Part model, mm, in its own coordinate system. A direction names the side the tool comes from. Coordinates: 2 decimals unless noted, no trailing zeros. Order: outer loops, then holes, each group sorted by start corner. A loop starts at its lowest first (then second) coordinate and runs counter-clockwise, first axis right, second up.
1) Wall check: L1, parallel to Y at x = -169.5, z = 124; L2, parallel to X at y = 385, z = 123.75; L3, parallel to Z at x = -194.65, y = 350.7. Give the ranges that are in metal, low to high.
2) Mould opens along Z. For faces 6 (the cylindrical face through (-194.72, 349, 132.57)), 7 (the flat face through (-177, 367, 117.5)), 8 (the cylindrical face through (-175.88, 368.68, 116.02)) say: +Z half, -Z half, draft (parallel to the pull), parting line (faces both ways), or undercut.
3) Pin check, flat tips, straight feed: pin 1 Ø5 at (x, z) = (-184, 130.5) entering from -Y; pin 2 Ø6 at (x, y) = (-160, 388.5) entering from +Z; pin 3 Ø8 at (x, z) = (-152, 126.5) entering from +Y; pin 4 Ø12 at (x, z) = (-172.5, 125) entering from -Y. Stop position of each tip, or through.
4) Tool access for faces 1 (the flat face through (-190, 363, 140.405)), 2 (the flat face through (-165, 379, 129.5)), 3 (the flat face through (-193, 386, 134)), 4 (the cylindrical face through (-153.436, 344.674, 121.049)), 5 (the flat face through (-191, 370.7, 134)): list every direction of +Z, -Z, +X, -X, +Y, -Y with a clear straight run to the whole face (end or side of a thin tool).
5) Cut at B-B (y = 383.7). Give the number of separate pieces and of enclosed holes in the cut face, and give its area (3 significant figures).
6) Cut at A-A (z = 127). List the corners of the cut face in (x, y), and give its area (3 significant figures).
```python
from build123d import *

# Parameters (mm, degrees)
BOX_W           = 55
BOX_H           = 95
BOX_DEPTH       = 10
SKETCH_R        = 2
POCKET_DEPTH    = 10
SKETCH001_R     = 2
POCKET001_DEPTH = 10
FILLET_R        = 1
PAD_DEPTH       = 20
CHAMFER_SIZE    = 20
CHAMFER001_SIZE = 20
SKETCH003_R     = 3
POCKET005_DEPTH = 6
SKETCH004_R     = 10
SKETCH004_R_2   = 2
PAD001_DEPTH    = 5
SKETCH005_W     = 3
SKETCH005_H     = 3
POCKET006_DEPTH = 5
SKETCH006_R     = 2.9
POCKET007_DEPTH = 3.5
SKETCH007_R     = 1.7
POCKET008_DEPTH = 5
SKETCH009_R     = 4.8
POCKET009_DEPTH = 9.5
CHAMFER002_SIZE = 1
CHAMFER003_SIZE = 1.5
SKETCH010_R     = 1.5
POCKET010_DEPTH = 8
SKETCH011_R     = 3
POCKET011_DEPTH = 1


with BuildPart() as part:
    # Box → Box (new body)
    with BuildSketch(Plane(origin=(-197, 315.2, 114.5), x_dir=(1, 0, 0), z_dir=(0, 0, 1))):
        with Locations((27.5, 47.5)):
            Rectangle(BOX_W, BOX_H)
    extrude(amount=BOX_DEPTH)

    # Sketch → Pocket (cut)
    with BuildSketch(Plane(origin=(-197, 315.2, 124.5), x_dir=(1, 0, 0), z_dir=(0, 0, 1))):
        with Locations((27.5, 26.5)):
            Circle(SKETCH_R)
        with Locations((27.5, 68.5)):
            Circle(SKETCH_R)
        Polygon((0, 74), (21.746137, 95), (0, 95), align=None)
        Polygon((33.253863, 95), (55, 95), (55, 74), align=None)
        Polygon((55, 21), (33.253863, 0), (55, 0), align=None)
        Polygon((0, 21), (0, 0), (21.746137, 0), align=None)
    extrude(amount=-POCKET_DEPTH, mode=Mode.SUBTRACT)

    # Sketch001 → Pocket001 (cut)
    with BuildSketch(Plane(origin=(-197, 315.2, 124.5), x_dir=(1, 0, 0), z_dir=(0, 0, 1))):
        with Locations((19.272759, 12.25)):
            Circle(SKETCH001_R)
        with Locations((19.272759, 40.75)):
            Circle(SKETCH001_R)
        with Locations((43.954483, 26.5)):
            Circle(SKETCH001_R)
        with Locations((19.272759, 54.25)):
            Circle(SKETCH001_R)
        with Locations((19.272759, 82.75)):
            Circle(SKETCH001_R)
        with Locations((43.954483, 68.5)):
            Circle(SKETCH001_R)
        with BuildLine():
            ThreePointArc((14.272759, 41.501336), (7.5, 26.5), (14.272759, 11.498664))
            Line((14.272759, 11.498664), (14.272759, 41.501336))
        make_face()
        with BuildLine():
            ThreePointArc((14.272759, 83.501336), (7.5, 68.5), (14.272759, 53.498664))
            Line((14.272759, 53.498664), (14.272759, 83.501336))
        make_face()
    extrude(amount=-POCKET001_DEPTH, mode=Mode.SUBTRACT)

    # Fillet
    fillet_edges = [part.edges().sort_by_distance(p)[0] for p in [
        (-182.727241, 326.698664, 119.5),
        (-175.727241, 355.95, 119.5),
        (-175.727241, 397.95, 119.5),
        (-182.727241, 356.701336, 119.5),
    ]]
    fillet(fillet_edges, radius=FILLET_R)

    # Sketch002 → Pad (new body)
    with BuildSketch(Plane(origin=(-197, 315.2, 124.5), x_dir=(1, 0, 0), z_dir=(0, 0, 1))):
        Polygon((4, 17.137245), (4, 31.5), (8, 31.5), (8, 39.5), (4, 39.5), (4, 45.5), (55, 45.5), (55, 49.5), (4, 49.5), (4, 55.5), (8, 55.5), (8, 63.5), (4, 63.5), (4, 77.862755), (0, 74), (0, 21), align=None)
    extrude(amount=PAD_DEPTH)

    # Chamfer
    chamfer_edges = [part.edges().sort_by_distance(p)[0] for p in [
        (-142, 362.7, 144.5),
    ]]
    chamfer(chamfer_edges, length=CHAMFER_SIZE)

    # Chamfer001
    chamfer001_edges = [part.edges().sort_by_distance(p)[0] for p in [
        (-162, 362.7, 144.5),
    ]]
    chamfer(chamfer001_edges, length=CHAMFER001_SIZE)

    # Sketch003 → Pocket005 (cut)
    with BuildSketch(Plane(origin=(-197, 315.2, 124.5), x_dir=(1, 0, 0), z_dir=(0, 0, 1))):
        with Locations((19.272759, 40.75)):
            Circle(SKETCH003_R)
        with Locations((19.272759, 12.25)):
            Circle(SKETCH003_R)
        with Locations((43.954483, 26.5)):
            Circle(SKETCH003_R)
        with Locations((19.272759, 54.25)):
            Circle(SKETCH003_R)
        with Locations((19.272759, 82.75)):
            Circle(SKETCH003_R)
        with Locations((43.954483, 68.5)):
            Circle(SKETCH003_R)
    extrude(amount=-POCKET005_DEPTH, mode=Mode.SUBTRACT)

    # Sketch004 → Pad001 (new body)
    with BuildSketch(Plane(origin=(-197, 315.2, 124.5), x_dir=(1, 0, 0), z_dir=(0, 0, 1))):
        with Locations((27.5, 68.5)):
            Circle(SKETCH004_R)
        with Locations((27.5, 68.5)):
            Circle(SKETCH004_R_2, mode=Mode.SUBTRACT)
        with Locations((27.5, 26.5)):
            Circle(SKETCH004_R)
        with Locations((27.5, 26.5)):
            Circle(SKETCH004_R_2, mode=Mode.SUBTRACT)
    extrude(amount=PAD001_DEPTH)

    # Sketch005 → Pocket006 (cut)
    with BuildSketch(Plane(origin=(-197, 360.7, 114.5), x_dir=(1, 0, 0), z_dir=(0, -1, 0))):
        with Locations((7.05428, 24.404704)):
            Rectangle(SKETCH005_W, SKETCH005_H)
        with Locations((20.05428, 24.404704)):
            Rectangle(SKETCH005_W, SKETCH005_H)
    extrude(amount=-POCKET006_DEPTH, mode=Mode.SUBTRACT)

    # Sketch006 → Pocket007 (cut)
    with BuildSketch(Plane(origin=(-189, 315.2, 114.5), x_dir=(0, 1, 0), z_dir=(1, 0, 0))):
        with Locations((35.5, 18)):
            Circle(SKETCH006_R)
        with Locations((59.5, 18)):
            Circle(SKETCH006_R)
    extrude(amount=-POCKET007_DEPTH, mode=Mode.SUBTRACT)

    # Sketch007 → Pocket008 (cut)
    with BuildSketch(Plane(origin=(-192.5, 315.2, 114.5), x_dir=(0, 1, 0), z_dir=(1, 0, 0))):
        with Locations((35.5, 18)):
            Circle(SKETCH007_R)
        with Locations((59.5, 18)):
            Circle(SKETCH007_R)
    extrude(amount=-POCKET008_DEPTH, mode=Mode.SUBTRACT)

    # Sketch009 → Pocket009 (cut)
    with BuildSketch(Plane(origin=(-197, 315.2, 129.5), x_dir=(1, 0, 0), z_dir=(0, 0, 1))):
        with Locations((27.5, 26.5)):
            Circle(SKETCH009_R)
        with Locations((27.5, 68.5)):
            Circle(SKETCH009_R)
    extrude(amount=-POCKET009_DEPTH, mode=Mode.SUBTRACT)

    # Chamfer002
    chamfer002_edges = [part.edges().sort_by_distance(p)[0] for p in [
        (-174.3, 383.7, 129.5),
        (-174.3, 341.7, 129.5),
    ]]
    chamfer(chamfer002_edges, length=CHAMFER002_SIZE)

    # Chamfer003
    chamfer003_edges = [part.edges().sort_by_distance(p)[0] for p in [
        (-171.5, 341.7, 120),
        (-171.5, 383.7, 120),
    ]]
    chamfer(chamfer003_edges, length=CHAMFER003_SIZE)

    # Sketch010 → Pocket010 (cut)
    with BuildSketch(Plane(origin=(-142, 315.2, 114.5), x_dir=(0, 1, 0), z_dir=(1, 0, 0))):
        with Locations((30, 5)):
            Circle(SKETCH010_R)
        with Locations((65, 5)):
            Circle(SKETCH010_R)
    extrude(amount=-POCKET010_DEPTH, mode=Mode.SUBTRACT)

    # Sketch011 → Pocket011 (cut)
    with BuildSketch(Plane(origin=(-197, 315.2, 118.5), x_dir=(1, 0, 0), z_dir=(0, 0, 1))):
        with Locations((19.272759, 82.75)):
            Circle(SKETCH011_R)
        with Locations((43.954483, 68.5)):
            Circle(SKETCH011_R)
        with Locations((19.272759, 54.25)):
            Circle(SKETCH011_R)
        with Locations((19.272759, 40.75)):
            Circle(SKETCH011_R)
        with Locations((43.954483, 26.5)):
            Circle(SKETCH011_R)
        with Locations((19.272759, 12.25)):
            Circle(SKETCH011_R)
    extrude(amount=-POCKET011_DEPTH, mode=Mode.SUBTRACT)


solid = part.part
```
Geometry check:
1. L1: y = 315.2 to 336.9, 346.5 to 378.9, 388.5 to 410.2
1. L2: x = -197 to -189.46, -182.73 to -174.12, -164.88 to -155.75, -150.34 to -142
1. L3: z = 114.5 to 130.8, 134.2 to 144.5
2. face 6: undercut
2. face 7: +Z half
2. face 8: draft
3. pin 1: stops at y = 360.7
3. pin 2: stops at z = 129.5
3. pin 3: stops at y = 402.2
3. pin 4: stops at y = 315.2
4. face 1: none
4. face 2: +Z, +X, +Y
4. face 3: +Z, +Y
4. face 4: +Z
4. face 5: +Z, +X
5. separate pieces: 4
5. enclosed holes: 0
5. area: 492 mm2
6. outline: (-197, 336.2) - (-193, 332.34) - (-193, 346.7) - (-189, 346.7) - (-189, 354.7) - (-193, 354.7) - (-193, 360.7) - (-144.5, 360.7) - (-144.5, 364.7) - (-193, 364.7) - (-193, 370.7) - (-189, 370.7) - (-189, 378.7) - (-193, 378.7) - (-193, 393.06) - (-197, 389.2) - close; circle Ø20 at (-169.5, 341.7); circle Ø20 at (-169.5, 383.7); hole circle Ø9.6 at (-169.5, 341.7); hole circle Ø9.6 at (-169.5, 383.7)
6. area: 969 mm2
